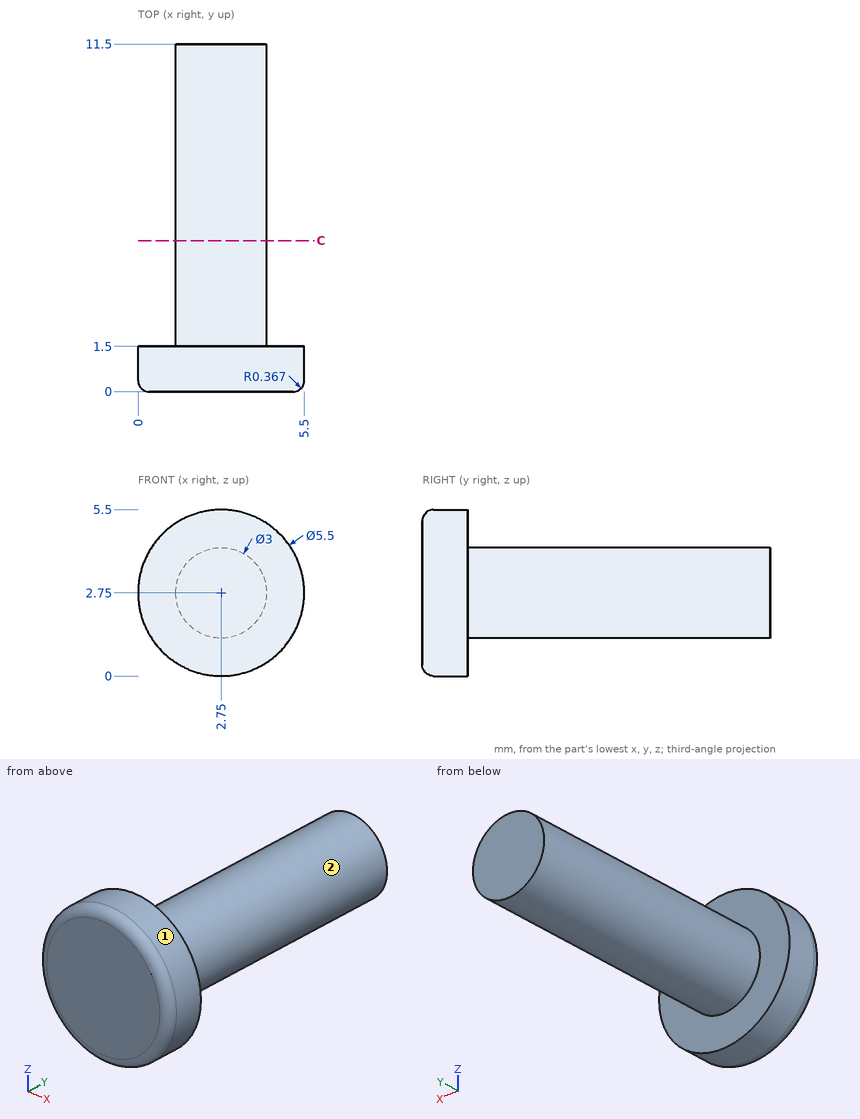
Geometry: see drawing. Coordinates: mm, zero at the bounding-box minimum. A direction names the side the tool comes from. Coordinates: 2 decimals unless noted, no trailing zeros. Order: outer loops, then holes, each group sorted by start corner. A loop starts at its lowest first (then second) coordinate and runs counter-clockwise, first axis right, second up. Notation, with made-up numbers: (39, 82.25) - (74, 82.25) arc R20 cw to (74, 91.25) - close; hole circle Ø9 at (52.25, 39). An arc over 180 degrees is marked (long way). Return JSON: item names as keys, results as strings.
Q1. First-contact query: pin 1 (1 mm diameter, centred on x = 4.5, z = 4.5, fed in from +Y). Flat tip, straight axial feed; report the tip coordinate or a pass-through.
The answers:
{"pin 1": "stops at y = 1.5"}
Q2. Access query for the marked faces 1 and 2. Directions: +Z, -Z, +X, -X, +Y, -Y. A direction counts if a zero-diameter tool reaches every point of the face in a straight line with its end or side. Return the directions, or none.
The answers:
{"face 1": "+Y, -Y", "face 2": "+Y"}
Q3. Ray query, probe 1 along X at (y, z) = (4.5, 2.8); probe 2 along Y at (x, z) = (0.55, 2.6). Return the intervals inside material, ascending.
The answers:
{"probe 1": "x = 1.25 to 4.25", "probe 2": "y = 0 to 1.5"}
Q4. Cut plane C-C (y = 5). Return loops of the section in (x, z).
The answers:
{"outline": "circle Ø3 at (2.75, 2.75)"}
